```python
from build123d import *

# Parameters (mm, degrees)
SKETCH003_W     = 36
SKETCH003_H     = 2
PAD_DEPTH       = 2
SKETCH004_R     = 0.65
POCKET001_DEPTH = 5
FILLET_R        = 0.7


with BuildPart() as part:
    # Sketch003 → Pad (new body)
    with BuildSketch(Plane.XY):
        with Locations((18, -1)):
            Rectangle(SKETCH003_W, SKETCH003_H)
    extrude(amount=PAD_DEPTH)

    # Sketch004 (on Face6 of Pad) → Pocket001 (cut)
    with BuildSketch(Plane.XY.offset(2)):
        with Locations((2, -1)):
            Circle(SKETCH004_R)
        with Locations((34, -1)):
            Circle(SKETCH004_R)
    extrude(amount=-POCKET001_DEPTH, mode=Mode.SUBTRACT)

    # Fillet
    fillet_edges = [part.edges().sort_by_distance(p)[0] for p in [
        (0, 0, 1),
        (0, -2, 1),
        (36, -2, 1),
        (36, 0, 1),
    ]]
    fillet(fillet_edges, radius=FILLET_R)


solid = part.part
```
Check sheet for the modelled part. Datum: model origin and axes. Units: mm. Coordinates: 2 decimals unless noted, no trailing zeros. Write each loop counter-clockwise with the first axis right and the second up, starting at its lowest first coordinate (ties: lowest second). Pieces come first, ordered by that corner, then holes. Notation, with made-up numbers: (66, 46.5) -> (125, 46.5) arc R22 cw to (125, 80.5) -> close; hole circle Ø10 at (17.5, -12.5). An arc over 180 degrees is marked (long way). Use a Markdown table: item, result.
1. Sectioned sample at C-C (y = -1). Enter the section's corners in (x, z).
Reported:
| item | result |
|---|---|
| outline | (0, 0) -> (1.35, 0) -> (1.35, 2) -> (0, 2) -> close; (2.65, 0) -> (33.35, 0) -> (33.35, 2) -> (2.65, 2) -> close; (34.65, 0) -> (36, 0) -> (36, 2) -> (34.65, 2) -> close |
2. Sectioned sample at B-B (z = 0.4). Enter the section's corners in (x, y).
Reported:
| item | result |
|---|---|
| outline | (0, -1.3) arc R0.7 ccw to (0.7, -2) -> (35.3, -2) arc R0.7 ccw to (36, -1.3) -> (36, -0.7) arc R0.7 ccw to (35.3, 0) -> (0.7, 0) arc R0.7 ccw to (0, -0.7) -> close; hole circle Ø1.3 at (2, -1); hole circle Ø1.3 at (34, -1) |
3. Release check for a two-part mould opening along Y. For faces 1 (the flat face through (18, -1, 2)), 2 (the flat face through (18, 0, 1)), 3 (the cylindrical face through (34.6, -1.25, 1.01)) record: pulls with the +Y half, pulls with the -Y half, needs draft (parallel to the pull), parting line crosses it, or undercut.
Reported:
| item | result |
|---|---|
| face 1 | needs draft |
| face 2 | pulls with the +Y half |
| face 3 | undercut |
4. Sectioned sample at A-A (x = 34). Enter the section's corners in (y, z).
Reported:
| item | result |
|---|---|
| outline | (-2, 0) -> (-1.65, 0) -> (-1.65, 2) -> (-2, 2) -> close; (-0.35, 0) -> (0, 0) -> (0, 2) -> (-0.35, 2) -> close |
5. Scan lines: line 1 along Y through (x, z) = (2, 0.9); line 2 along X through (y, z) = (-0.9, 0.8); line 3 along X through (y, z) = (-1.35, 0.3). Record each from-to range of solid material in increasing order.
Reported:
| item | result |
|---|---|
| line 1 | y = -2 to -1.65, -0.35 to 0 |
| line 2 | x = 0 to 1.36, 2.64 to 33.36, 34.64 to 36 |
| line 3 | x = 0 to 1.45, 2.55 to 33.45, 34.55 to 36 |
